Model file for the job. Use its own axes, mm. A direction names the side the tool comes from. Round coordinates to 2 decimals unless told otherwise and drop trailing zeros. Order: outer loops, then holes, each group sorted by start corner. A loop starts at its lowest first (then second) coordinate and runs counter-clockwise, first axis right, second up. Notation, with made-up numbers: (83.5, -30) -> (98.5, -30) arc R16 cw to (98.5, -19) -> close; hole circle Ø7 at (-0.75, -20.75). An arc over 180 degrees is marked (long way). Use CSV: the item, a comma, the result in double quotes.
```python
from build123d import *

# Parameters (mm, degrees)
SKETCH1_W                     = 99
SKETCH1_H                     = 60
BOSS_EXTRUDE1_DEPTH           = 4
CBORE_FOR_M3_SHCS1_AT_2_COUNT = 2
CBORE_FOR_M3_SHCS1_AT_2_PITCH = 20
M3X0_5_TAPPED_HOLE1_D         = 2.5


with BuildPart() as part:
    # Sketch1 → Boss-Extrude1 (new body, symmetric)
    with BuildSketch(Plane.XY):
        Rectangle(SKETCH1_W, SKETCH1_H)
    extrude(amount=BOSS_EXTRUDE1_DEPTH, both=True)

    # Sketch3 → CBORE for M3 SHCS1 (revolve, cut)
    with BuildSketch(Plane(origin=(-42, 10, 4), x_dir=(0, -1, 0), z_dir=(1, 0, 0))):
        Polygon((0, 0), (0, 8), (1.725, 8), (1.7, 7.975), (1.7, 3), (3.25, 3), (3.25, 0.025), (3.275, 0), align=None)
    cbore_for_m3_shcs1 = revolve(axis=Axis((-42, 10, 10.35), (0, 0, -1)), mode=Mode.SUBTRACT)

    # CBORE for M3 SHCS1 at 2: CBORE for M3 SHCS1 ×2
    with Locations(*[(0, -i * CBORE_FOR_M3_SHCS1_AT_2_PITCH, 0) for i in range(1, CBORE_FOR_M3_SHCS1_AT_2_COUNT)]):
        add(cbore_for_m3_shcs1, mode=Mode.SUBTRACT)

    # M3x0.5 Tapped Hole1 (through all)
    with Locations(Plane.XY.offset(4)):
        with Locations((-23.5, -0.8)):
            m3x0_5_tapped_hole1 = Hole(M3X0_5_TAPPED_HOLE1_D / 2)

    # Mirror1: M3x0.5 Tapped Hole1, CBORE for M3 SHCS1 across plane
    add(m3x0_5_tapped_hole1.mirror(Plane(origin=(0, 0, 0), x_dir=(0, 0, 1), z_dir=(1, 0, 0))), mode=Mode.SUBTRACT)
    add(cbore_for_m3_shcs1.mirror(Plane(origin=(0, 0, 0), x_dir=(0, 0, 1), z_dir=(1, 0, 0))), mode=Mode.SUBTRACT)

    # Mirror1 copy 1 sketch → Mirror1 copy 1 (revolve, cut)
    with BuildSketch(Plane(origin=(42, -10, 4), x_dir=(0, -1, 0), z_dir=(-1, 0, 0))):
        Polygon((0, 0), (0, -8), (1.725, -8), (1.7, -7.975), (1.7, -3), (3.25, -3), (3.25, -0.025), (3.275, 0), align=None)
    revolve(axis=Axis((42, -10, 10.35), (0, 0, 1)), mode=Mode.SUBTRACT)


solid = part.part
```
Q1. Probe line 1 along X through (y, z) = (10, 1.95); line 2 along Y through (x, z) = (-42, 0.25); line 3 along X through (y, z) = (10, -1.4). List the from-to ranges inside material, lowest first.
From the geometry:
line 1,"x = -49.5 to -45.25, -38.75 to 38.75, 45.25 to 49.5"
line 2,"y = -30 to -11.7, -8.3 to 8.3, 11.7 to 30"
line 3,"x = -49.5 to -43.7, -40.3 to 40.3, 43.7 to 49.5"
Q2. Mould opens along X. For faces 1 (the cylindrical face through (24.69, -0.42, -0.06)), 2 (the flat face through (-1, 0, -4)), 3 (the flat face through (49.5, 0, 0)), 4 (the flat face through (-40.6, 11.4, 1)) say: +X half, -X half, draft (parallel to the pull), parting line (faces both ways), or undercut.
From the geometry:
face 1,"undercut"
face 2,"draft"
face 3,"+X half"
face 4,"undercut"
Q3. Cut at B-B (x = 23.5). Give the cut face in (y, z).
From the geometry:
outline,"(-30, -4) -> (-2.05, -4) -> (-2.05, 4) -> (-30, 4) -> close; (0.45, -4) -> (30, -4) -> (30, 4) -> (0.45, 4) -> close"
Q4. Pin check, flat tips, straight feed: pin 1 (5 mm diameter, centred on x = 42, y = 10, fed in from +Z); pin 2 (3 mm diameter, centred on x = -42, y = -10, fed in from +Z). Stop position of each tip, or through.
From the geometry:
pin 1,"stops at z = 1"
pin 2,"passes through"
Q5. Cut at A-A (y = -0.8). Give the cut face in (x, z), plus the area to 3 significant figures.
From the geometry:
outline,"(-49.5, -4) -> (-24.75, -4) -> (-24.75, 4) -> (-49.5, 4) -> close; (-22.25, -4) -> (22.25, -4) -> (22.25, 4) -> (-22.25, 4) -> close; (24.75, -4) -> (49.5, -4) -> (49.5, 4) -> (24.75, 4) -> close"
area,"752 mm²"
Q6. Which spindle directions (+Z, -Z, +X, -X, +Y, -Y) get a long thin tool onto all of the face, cutting with end or side? Do faces 5 (the cylindrical face through (38.827, 10.705, 2.508)), 6 (the flat face through (-1, 30, 0)). Say none if no direction does.
From the geometry:
face 5,"+Z"
face 6,"+Z, -Z, +X, -X, +Y"
Q7. Cut at C-C (x = -42). Give the cut face in (y, z) (3 decimals).
From the geometry:
outline,"(-30, -4) -> (-11.725, -4) -> (-11.7, -3.975) -> (-11.7, 1) -> (-13.25, 1) -> (-13.25, 3.975) -> (-13.275, 4) -> (-30, 4) -> close; (-8.3, -3.975) -> (-8.275, -4) -> (8.275, -4) -> (8.3, -3.975) -> (8.3, 1) -> (6.75, 1) -> (6.75, 3.975) -> (6.725, 4) -> (-6.725, 4) -> (-6.75, 3.975) -> (-6.75, 1) -> (-8.3, 1) -> close; (11.7, -3.975) -> (11.725, -4) -> (30, -4) -> (30, 4) -> (13.275, 4) -> (13.25, 3.975) -> (13.25, 1) -> (11.7, 1) -> close"
